The figure shows three views and two pictorial views of one solid part (mm, origin at its lowest corner). Answer the questions. Give positions to 0.01 mm unless a question says otherwise; leave off trailing zeros. Write each loop counter-clockwise with the first axis right and the second up, starting at its lowest first coordinate (ties: lowest second). Pieces come first, ordered by that corner, then holes. Notation, with made-up numbers: (32, 52) - (45, 52) arc R25 cw to (45, 83) - close; hole circle Ø11 at (-26.75, 16). An arc over 180 degrees is marked (long way). One line per question, with ' | ' between items. Start each with the question number.
1. A cutting plane is placed at D-D (z = 19.5). Determine the outline of the cut face in (x, y), then the cut area to 3 significant figures.
2. A cutting plane is placed at C-C (y = 3). State how many separate pieces and enclosed holes the cut face has, then the cut area to 3 significant figures.
3. A cutting plane is placed at A-A (z = 15). Determine the outline of the cut face in (x, y), then the cut area to 3 significant figures.
4. A cutting plane is placed at B-B (x = 42.5). Determine the outline of the cut face in (y, z).
5. Find the intervals of material crossed by L1, parallel to X at y = 3, z = 15; L2, parallel to Z at x = 39.5, y = 4.5; L3, parallel to X at y = 2.25, z = 3.75, in increasing order. Write a range as from..to.
6. The mould has two halves that part along Z. Classify the marked faces 1, 2 and 3: +Z half, -Z half, draft (parallel to the pull), parting line (faces both ways), or undercut.
7. Given P1, Ø1.5, axis at y = 3.5, z = 27, coming from the +X side; P2, Ø1, axis at x = 50, z = 4, coming from the -Y side; P3, Ø3.5, axis at x = 42.5, z = 26.5, coming from the +Y side, each flat-ended and moving along its own axis, determine where each tip first touches the part or whether it passes through.
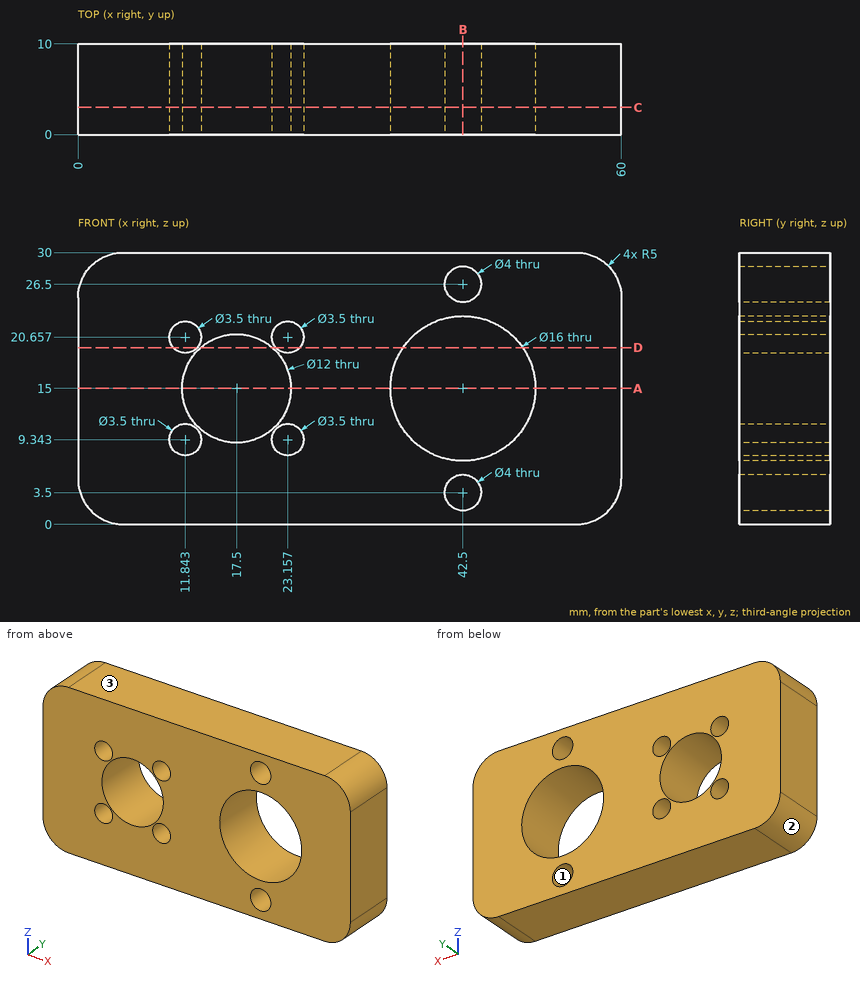
Determined:
1) outline: (0, 0) - (10.53, 0) - (10.53, 10) - (0, 10) - close; (13.16, 0) - (13.53, 0) - (13.53, 10) - (13.16, 10) - close; (21.47, 0) - (21.84, 0) - (21.84, 10) - (21.47, 10) - close; (24.47, 0) - (35.89, 0) - (35.89, 10) - (24.47, 10) - close; (49.11, 0) - (60, 0) - (60, 10) - (49.11, 10) - close | area: 336 mm2
2) separate pieces: 1 | enclosed holes: 8 | area: 1,400 mm2
3) outline: (0, 0) - (11.5, 0) - (11.5, 10) - (0, 10) - close; (23.5, 0) - (34.5, 0) - (34.5, 10) - (23.5, 10) - close; (50.5, 0) - (60, 0) - (60, 10) - (50.5, 10) - close | area: 320 mm2
4) outline: (0, 0) - (10, 0) - (10, 1.5) - (0, 1.5) - close; (0, 5.5) - (10, 5.5) - (10, 7) - (0, 7) - close; (0, 23) - (10, 23) - (10, 24.5) - (0, 24.5) - close; (0, 28.5) - (10, 28.5) - (10, 30) - (0, 30) - close
5) L1: 0..11.5, 23.5..34.5, 50.5..60 | L2: 0..7.58, 22.42..30 | L3: 0.16..40.52, 44.48..59.84
6) face 1: undercut | face 2: -Z half | face 3: +Z half
7) P1: x = 59.84 | P2: y = 0 | P3: through
